Part model, mm, in its own coordinate system. Face numbers are marked on the shaded views. A direction names the side the tool comes from. Round coordinates to 2 decimals unless told otherwise and drop trailing zeros. Loops run counter-clockwise (first coordinate to the right, second up) from the corner with the lowest first, then second, coordinate; pieces in that order, holes last. Notation, with made-up numbers: (-2.75, -24) - (43.25, -24) arc R27 ccw to (43.25, -8) - close; hole circle Ø6 at (60, 20.5). An arc over 180 degrees is marked (long way). Write each question's results on one line, items separated by ' | '. Start each with the question number.
(1) Cut at A-A, the plane x = 28. List the corners of the cut face in (y, z).
(2) Tool access for the marked faces 1, 2 and 3: list every direction of +Z, -Z, +X, -X, +Y, -Y with a clear straight run to the whole face (end or side of a thin tool).
(3) Cut at B-B, the plane z = 90.5. List the corners of the cut face in (x, y).
(4) Cut at C-C, the plane x = 79. List the corners of the cut face in (y, z).
(5) Flat gauge pins, fed straight in: P1, Ø6, axis at y = 8.5, z = 24, coming from the +X side; P2, Ø1.5, axis at x = 11, y = 3.5, coming from the -Z side; P3, Ø2, axis at x = 76, y = 6, coming from the +Z side; P4, Ø1.5, axis at x = 167.5, y = 3.5, coming from the -Z side. Where does each tip first touch, or does it go through?
(6) Drill centre lines: L1, parallel to Y at x = 159.5, z = 150; L2, parallel to Z at x = 106, y = 4; L3, parallel to X at y = 1.35, z = 162. Where is each one in solid material? Low to high.
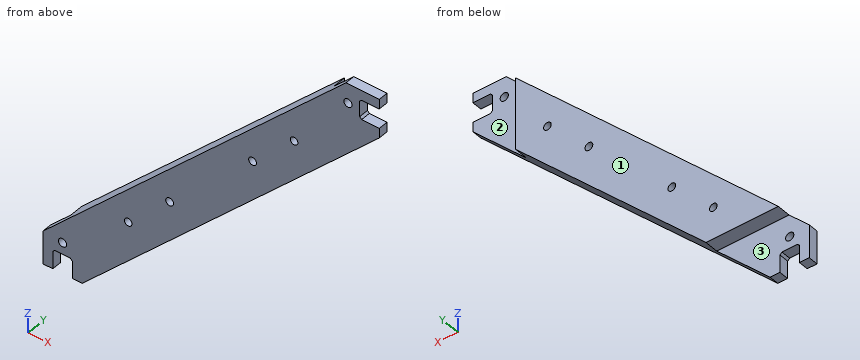
from build123d import *

# Parameters (mm, degrees)
MAIN_BASE_EXTRUDE_DEPTH       = 12
SKETCH3_W                     = 47.3
SKETCH3_H                     = 27.3
SKETCH3_W_2                   = 27.3
SKETCH3_H_2                   = 47.3
TRACK_SEAT_CUT_DEPTH          = 7
SKETCH2_R                     = 2.1
TRACK_CONNECT_HOLES_DEPTH     = 244.540551038
WALL_SPACED_HOLES_DEPTH       = 244.540551038
WALL_SPACED_HOLES_DEPTH_BACK  = 244.540551038
SKETCH5_R                     = 1.95
SKETCH5_R_2                   = 2
SKETCH9_W                     = 10
SKETCH9_H                     = 10
WIRE_PASSTHROUGH_CUT_DEPTH    = 244.345433489
WIRE_PASSTHROUGH_CHAMFER_SIZE = 1


with BuildPart() as part:
    # Sketch1 → Main Base Extrude (new body)
    with BuildSketch(Plane(origin=(0, 0, 0), x_dir=(1, 0, 0), z_dir=(0, 1, 0))):
        Polygon((0, 0), (20, 0), (172, -152), (172, -172), (155, -172), (0, -17), align=None)
    extrude(amount=MAIN_BASE_EXTRUDE_DEPTH)

    # Sketch3 → Track Seat Cut (cut)
    with BuildSketch(Plane(origin=(0, 12, 0), x_dir=(1, 0, 0), z_dir=(0, 1, 0))):
        with Locations((23.65, -13.65)):
            Rectangle(SKETCH3_W, SKETCH3_H)
        with Locations((158.35, -148.35)):
            Rectangle(SKETCH3_W_2, SKETCH3_H_2)
    extrude(amount=-TRACK_SEAT_CUT_DEPTH, mode=Mode.SUBTRACT)

    # Sketch2 → Track Connect Holes (cut, through all)
    with BuildSketch(Plane(origin=(0, 12, 0), x_dir=(1, 0, 0), z_dir=(0, 1, 0))):
        with Locations(Location((10, -16, 0), (0, 0, 270))):
            Circle(SKETCH2_R)
        with Locations(Location((156, -162, 0), (0, 0, 270))):
            Circle(SKETCH2_R)
    extrude(amount=-TRACK_CONNECT_HOLES_DEPTH, mode=Mode.SUBTRACT)

    # Sketch5 → Wall Spaced Holes (cut, two sides: drawn at the far end of the back side and taken through both)
    with BuildSketch(Plane(origin=(0, 0, 0), x_dir=(1, 0, 0), z_dir=(0, 1, 0)).offset(-WALL_SPACED_HOLES_DEPTH_BACK)):
        with Locations(Location((128.411688245, -128.441125497, 0), (0, 0, 270))):
            Circle(SKETCH5_R)
        with Locations(Location((107.19848481, -107.227922061, 0), (0, 0, 270))):
            Circle(SKETCH5_R_2)
        with Locations(Location((43.558874503, -43.588311755, 0), (0, 0, 90))):
            Circle(SKETCH5_R)
        with Locations(Location((64.772077939, -64.80151519, 0), (0, 0, 90))):
            Circle(SKETCH5_R_2)
    extrude(amount=WALL_SPACED_HOLES_DEPTH + WALL_SPACED_HOLES_DEPTH_BACK, mode=Mode.SUBTRACT)

    # Sketch9 → Wire Passthrough Cut (cut, through all)
    with BuildSketch(Plane(origin=(0, 5, 0), x_dir=(1, 0, 0), z_dir=(0, 1, 0))):
        with Locations((10, -5)):
            Rectangle(SKETCH9_W, SKETCH9_H)
        with Locations((167, -162)):
            Rectangle(SKETCH9_W, SKETCH9_H)
    extrude(amount=-WIRE_PASSTHROUGH_CUT_DEPTH, mode=Mode.SUBTRACT)

    # Wire Passthrough Chamfer
    wire_passthrough_chamfer_edges = [part.edges().sort_by_distance(p)[0] for p in [
        (5, 2.5, 10),
        (15, 2.5, 10),
        (162, 2.5, 167),
        (162, 2.5, 157),
    ]]
    chamfer(wire_passthrough_chamfer_edges, length=WIRE_PASSTHROUGH_CHAMFER_SIZE)


solid = part.part
A:
1) outline: (0, 8) - (5, 8) - (5, 27.3) - (12, 27.3) - (12, 45) - (0, 45) - close
2) face 1: +Z, -Z, +X, -X, +Y | face 2: +Z, -Z, +X, +Y | face 3: -Z, +X, -X, +Y
3) outline: (73.5, 0) - (110.5, 0) - (110.5, 12) - (73.5, 12) - close
4) outline: (0, 59) - (12, 59) - (12, 96) - (0, 96) - close
5) P1: through | P2: z = 10 | P3: z = 94 | P4: z = 146.75
6) L1: 0 to 5 | L2: 86 to 105.63, 108.83 to 123 | L3: 145 to 153.9, 158.1 to 162
